Read the model definition and answer for the solid it produces. Units are mm, in the model's axes. A direction names the side the tool comes from. Coordinates: 2 decimals unless noted, no trailing zeros. Write each loop counter-clockwise with the first axis right and the second up, starting at its lowest first coordinate (ties: lowest second). Pieces come first, ordered by that corner, then holes.
1) The part is cut by section C-C (x = -16). Give the number of separate pieces and of enclosed holes in the cut face, then the cut area to 3 significant figures.
2) The part is cut by section B-B (x = -12). Determine the outline of the cut face in (y, z), then the cut area to 3 significant figures.
3) Which of the six approach directions +Z, -Z, +X, -X, +Y, -Y give full straight-line access (tool end or side, diameter ignored) to faces 1 (the face through (-9, 4.15, 4)), 2 (the face through (0, 0, 0)), 3 (the face through (-9, 0, 6.9)), 4 (the face through (-14, -4, 0.31)), 5 (the face through (-9, -4.12, 4))?
4) Each of these flat-tipped pins is pushed along its axis until it touches: pin 1 Ø0.7 at (x, y) = (-17.5, 3.5) entering from -Z; pin 2 Ø0.5 at (x, y) = (-13.5, -3.5) entering from -Z; pin 3 Ø0.7 at (x, y) = (-17, -1.5) entering from +Z. Where does it stop, or does it pass through?
5) The part is cut by section D-D (x = 5.5). Determine the outline of the cut face in (y, z).
6) Find the intervals of material crossed by line 1 (Z direction, x = -20, y = 1.25); line 2 (Y direction, x = -15.5, z = 3.75); line 3 (Z direction, x = -5.5, y = -2.5), in increasing order.
7) The part is cut by section A-A (z = 3). Determine the outline of the cut face in (x, y), then the cut area to 3 significant figures.
Autodesk Fusion 360 part; units mm, degrees
sketch "Sketch1" plane through (0, 0, 0) normal (0, 0, 1) x (1, 0, 0)
  line L0 (-12.5, 5.5) -> (12.5, 5.5)
  line L1 (12.5, 5.5) -> (12.5, -5.5)
  line L2 (12.5, -5.5) -> (-12.5, -5.5)
  line L3 (-12.5, -5.5) -> (-12.5, 5.5)
  line L4 (-12.5, 5.5) -> (12.5, -5.5) construction
  line L5 (12.5, 5.5) -> (-12.5, -5.5) construction
  line L6 (-12.5, 5.5) -> (-21.5, 5.5) construction
  line L7 (-21.5, 5.5) -> (-21.5, -5.5) construction
  line L8 (-21.5, -5.5) -> (-12.5, -5.5) construction
  dimension "d1" = 11
  dimension "d2" = 25
  dimension "d5" = 34
extrude "Extrude1" add sketch "Sketch1" along normal blind 1 makes body 1
sketch "Sketch2" plane through (0, 0, 0) normal (0, 1, 0) x (1, 0, 0)
  line L0 (-15.25, -7.75) -> (-12.75, -7.75)
  line L1 (-12.75, -7.75) -> (-12.75, -0.31)
  line L2 (-12.75, -0.31) -> (-15.25, -0.31)
  line L3 (-15.25, -0.31) -> (-15.25, -7.75)
  point P0 (12.5, 0)
  dimension "d6" = 2.5
  dimension "d7" = 7.44
  dimension "d8" = 7.75
  dimension "d9" = 27.75
extrude "Extrude2" add sketch "Sketch2" along normal mid plane 10 separate body makes body 2
sketch "Sketch3" plane through (-15.25, 0, 0) normal (-1, 0, 0) x (0, -1, 0)
  line L0 (5, 7.75) -> (-5, 7.75)
  line L1 (-5, 7.75) -> (-5, 0.31)
  line L2 (-5, 0.31) -> (5, 0.31)
  line L3 (5, 0.31) -> (5, 7.75)
  line L4 (-4.15, 6.9) -> (-3.5, 6.9)
  line L5 (-3.5, 6.9) -> (-3.5, 6.25)
  line L6 (-3.5, 6.25) -> (-4.15, 6.25)
  line L7 (-4.15, 6.25) -> (-4.15, 6.9)
  line L8 (-1.61, 6.9) -> (-0.96, 6.9)
  line L9 (-0.96, 6.9) -> (-0.96, 6.25)
  line L10 (-0.96, 6.25) -> (-1.61, 6.25)
  line L11 (-1.61, 6.25) -> (-1.61, 6.9)
  line L12 (0.93, 6.9) -> (1.58, 6.9)
  line L13 (1.58, 6.9) -> (1.58, 6.25)
  line L14 (1.58, 6.25) -> (0.93, 6.25)
  line L15 (0.93, 6.25) -> (0.93, 6.9)
  line L16 (3.47, 6.9) -> (4.12, 6.9)
  line L17 (4.12, 6.9) -> (4.12, 6.25)
  line L18 (4.12, 6.25) -> (3.47, 6.25)
  line L19 (3.47, 6.25) -> (3.47, 6.9)
  line L20 (-4.15, 4.36) -> (-3.5, 4.36)
  line L21 (-3.5, 4.36) -> (-3.5, 3.71)
  line L22 (-3.5, 3.71) -> (-4.15, 3.71)
  line L23 (-4.15, 3.71) -> (-4.15, 4.36)
  line L24 (-1.61, 4.36) -> (-0.96, 4.36)
  line L25 (-0.96, 4.36) -> (-0.96, 3.71)
  line L26 (-0.96, 3.71) -> (-1.61, 3.71)
  line L27 (-1.61, 3.71) -> (-1.61, 4.36)
  line L28 (0.93, 4.36) -> (1.58, 4.36)
  line L29 (1.58, 4.36) -> (1.58, 3.71)
  line L30 (1.58, 3.71) -> (0.93, 3.71)
  line L31 (0.93, 3.71) -> (0.93, 4.36)
  line L32 (3.47, 4.36) -> (4.12, 4.36)
  line L33 (4.12, 4.36) -> (4.12, 3.71)
  line L34 (4.12, 3.71) -> (3.47, 3.71)
  line L35 (3.47, 3.71) -> (3.47, 4.36)
  line L36 (-4.15, 1.82) -> (-3.5, 1.82)
  line L37 (-3.5, 1.82) -> (-3.5, 1.17)
  line L38 (-3.5, 1.17) -> (-4.15, 1.17)
  line L39 (-4.15, 1.17) -> (-4.15, 1.82)
  line L40 (-1.61, 1.82) -> (-0.96, 1.82)
  line L41 (-0.96, 1.82) -> (-0.96, 1.17)
  line L42 (-0.96, 1.17) -> (-1.61, 1.17)
  line L43 (-1.61, 1.17) -> (-1.61, 1.82)
  line L44 (0.93, 1.82) -> (1.58, 1.82)
  line L45 (1.58, 1.82) -> (1.58, 1.17)
  line L46 (1.58, 1.17) -> (0.93, 1.17)
  line L47 (0.93, 1.17) -> (0.93, 1.82)
  line L48 (3.47, 1.82) -> (4.12, 1.82)
  line L49 (4.12, 1.82) -> (4.12, 1.17)
  line L50 (4.12, 1.17) -> (3.47, 1.17)
  line L51 (3.47, 1.17) -> (3.47, 1.82)
  line L52 (-5, 7) -> (-4.25, 7.75)
  line L53 (-3.21, 7.75) -> (-2.46, 7)
  line L54 (-2.46, 7) -> (-1.71, 7.75)
  line L55 (-0.75, 7.75) -> (0, 7)
  line L56 (0, 7) -> (0.7523, 7.7523)
  line L57 (1.71, 7.75) -> (2.46, 7)
  line L58 (2.46, 7) -> (3.21, 7.75)
  line L59 (4.25, 7.75) -> (5, 7)
  line L60 (-5, 7) -> (5, 7) construction
  line L61 (-5, 7) -> (-5, 8.8118)
  line L62 (-5, 8.8118) -> (5, 8.8118)
  line L63 (5, 8.8118) -> (5, 7)
  line L64 (-4.25, 7.75) -> (-3.21, 7.75)
  line L65 (-1.71, 7.75) -> (-0.75, 7.75)
  line L66 (0.7523, 7.7523) -> (1.71, 7.75)
  line L67 (3.21, 7.75) -> (4.25, 7.75)
  line L68 (-5, 1.06) -> (5, 1.06) construction
  line L69 (-5, 1.06) -> (-5, -0.1236)
  line L70 (-5, -0.1236) -> (5, -0.1236)
  line L71 (5, -0.1236) -> (5, 1.06)
  line L72 (5, 1.06) -> (4.25, 0.31)
  line L73 (4.25, 0.31) -> (3.21, 0.31)
  line L74 (3.21, 0.31) -> (2.46, 1.06)
  line L75 (2.46, 1.06) -> (1.71, 0.31)
  line L76 (1.71, 0.31) -> (0.75, 0.31)
  line L77 (0.75, 0.31) -> (0, 1.06)
  line L78 (0, 1.06) -> (-0.75, 0.31)
  line L79 (-0.75, 0.31) -> (-1.71, 0.31)
  line L80 (-1.71, 0.31) -> (-2.46, 1.06)
  line L81 (-2.46, 1.06) -> (-3.21, 0.31)
  line L82 (-3.21, 0.31) -> (-4.25, 0.31)
  line L83 (-4.25, 0.31) -> (-5, 1.06)
  line L84 (-4.15, 6.9) -> (4.12, 6.9)
  line L85 (4.12, 6.9) -> (4.12, 1)
  line L86 (4.12, 1) -> (-4.15, 1)
  line L87 (-4.15, 1) -> (-4.15, 6.9)
  line L88 (-5.5, 1) -> (5.5, 1)
  dimension "d12" = 0.65
  dimension "d13" = 0.65
  dimension "d16" = 2.54
  dimension "d17" = -2.54
  dimension "d18" = 0.85
  dimension "d19" = 0.85
  dimension "d20" = 0.75
  dimension "d21" = 90
  dimension "d22" = 45
  dimension "d23" = 90
  dimension "d24" = 90
  dimension "d25" = 45
  dimension "d26" = 2.54
  dimension "d27" = 2.54
  dimension "d28" = 0.75
extrude "Extrude3" cut sketch "Sketch3" against normal blind 3 contours L0 L3 L59 L63 | L0 L56 L61 L62 L63 L64 L65 L66 L67 | L0 L57 L58 | L3 L71 L72 L88 | L2 L3 L71 L72 L88 | L0 L1 L52 L61 | L0 L55 L56 | L2 L69 L70 L71 L73 L76 L79 L82 | L2 L74 L75 L86 L88 | L74 L75 L86 L88 | L0 L53 L54 | L1 L69 L83 L88 | L1 L2 L69 L83 L88 | L2 L77 L78 L86 L88 | L77 L78 L86 L88 | L2 L80 L81 L86 L88 | L80 L81 L86 L88 bodies 2
extrude "Extrude4" add sketch "Sketch3" along normal blind 6.14 contours L48 L49 L50 L51 L85 | L32 L33 L34 L35 L85 | L36 L37 L38 L39 L87 | L16 L17 L18 L19 L84 L85 | L20 L21 L22 L23 L87 | L12 L13 L14 L15 L84 | L4 L5 L6 L7 L84 L87 | L8 L9 L10 L11 L84 | L24 L25 L26 L27 | L28 L29 L30 L31 | L40 L41 L42 L43 | L44 L45 L46 L47 bodies 2
extrude "Extrude5" add sketch "Sketch3" against normal blind 7.36 from surface at -2.5 contours L5 L6 L9 L10 L11 L13 L14 L15 L18 L19 L20 L21 L22 L32 L34 L35 L36 L37 L38 L48 L50 L51 L74 L75 L77 L78 L80 L81 L84 L85 L86 L87 L88 | L48 L49 L50 L51 L85 | L74 L75 L86 L88 | L32 L33 L34 L35 L85 | L77 L78 L86 L88 | L80 L81 L86 L88 | L36 L37 L38 L39 L87 | L16 L17 L18 L19 L84 L85 | L20 L21 L22 L23 L87 | L12 L13 L14 L15 L84 | L4 L5 L6 L7 L84 L87 | L8 L9 L10 L11 L84 | L24 L25 L26 L27 | L28 L29 L30 L31 | L40 L41 L42 L43 | L44 L45 L46 L47 bodies 1 2
equation "d28 = d20"
Reported:
1. separate pieces: 12
1. enclosed holes: 0
1. area: 5.07 mm2
2. outline: (-5.5, 0) - (5.5, 0) - (5.5, 1) - (4.15, 1) - (4.15, 6.9) - (-4.12, 6.9) - (-4.12, 1) - (-5.5, 1) - close
2. area: 59.8 mm2
3. face 1: +Z, +X, +Y
3. face 2: -Z, +X, -X, +Y, -Y
3. face 3: +Z, +X, +Y, -Y
3. face 4: -Z, -X, +Y, -Y
3. face 5: +Z, +X, -Y
4. pin 1: stops at z = 1.17
4. pin 2: stops at z = 0.31
4. pin 3: stops at z = 6.9
5. outline: (-5.5, 0) - (5.5, 0) - (5.5, 1) - (-5.5, 1) - close
6. line 1: z = 1.17 to 1.82, 3.71 to 4.36, 6.25 to 6.9
6. line 2: y = -4.12 to -3.47, -1.58 to -0.93, 0.96 to 1.61, 3.5 to 4.15
6. line 3: z = 0 to 6.9
7. outline: (-15.25, -5) - (-12.75, -5) - (-12.75, -4.12) - (-5.39, -4.12) - (-5.39, 4.15) - (-12.75, 4.15) - (-12.75, 5) - (-15.25, 5) - close
7. area: 85.9 mm2
